Geometry: final body of the model. Coordinates: model frame, mm. A direction names the side the tool comes from. Give positions to 0.01 mm unless a question says otherwise; leave off trailing zeros. Order: outer loops, then holes, each group sorted by start corner. A loop starts at its lowest first (then second) coordinate and runs counter-clockwise, first axis right, second up. Notation, with made-up numbers: M -37.75,28 L 6.25,28 A11 cw 6.25,42 Z; hole C 74.25,68 d11. An arc over 180 degrees is marked long. Write item = value, one per line. Start each with the question number.
from build123d import *
from build123d.topology import SkipClean

# Parameters (mm, degrees)
BOSS_EXTRU_1_START = 5
BOSS_EXTRU_1_DEPTH = 5


with BuildPart() as part:
    # Esquisse1 → Révolution1 (revolve)
    with BuildSketch(Plane(origin=(0, 0, 0), x_dir=(1, 0, 0), z_dir=(0, 1, 0)), mode=Mode.PRIVATE) as r_volution1_sk:
        Polygon((-95.869703244, 5), (-95.869703244, -5), (-78.192033714, -22.67766953), (-78.192033714, -17.67766953), (-81, -14.869703244), (-81, 0), (-87.869703244, 0), (-87.869703244, 5), align=None)
    revolve(r_volution1_sk.sketch.rotate(Axis((0, 0, 0), (0, 0, -1)), 180), axis=Axis((0, 0, 0), (0, 0, -1)))

    # Esquisse6 → Boss.-Extru.1 (add)
    with SkipClean():  # the faces are left unmerged after this step: merging them gives an invalid solid
        with BuildSketch(Plane(origin=(0, 0, 0), x_dir=(-1, 0, 0), z_dir=(0, 0, -1)).offset(BOSS_EXTRU_1_START)):
            with BuildLine():
                Line((80.961410561, -2.5), (87.834132022, -2.5))
                ThreePointArc((87.834132022, -2.5), (87.869703244, 0), (87.834132022, 2.5))
                Line((87.834132022, 2.5), (80.961410561, 2.5))
                ThreePointArc((80.961410561, 2.5), (81, 0), (80.961410561, -2.5))
            make_face()
        boss_extru_1 = extrude(amount=-BOSS_EXTRU_1_DEPTH)

    # Symétrie1: Boss.-Extru.1 across plane
    add(boss_extru_1.mirror(Plane(origin=(0, 0, 0), x_dir=(0, 0, 1), z_dir=(1, 0, 0))))


solid = part.part
1) Cut plane B-B (y = 0). Return loops of the section in (x, z), plus the area to 3 significant figures.
2) Access query for faces 1 (the cylindrical face through (1.9, -87.85, -2.54)), 2 (the cylindrical face through (-20.78, 93.59, 0.07)). Directions: +Z, -Z, +X, -X, +Y, -Y. A direction counts if a zero-diameter tool reaches every point of the face in a straight line with its end or side. Return the directions, or none.
3) Cut plane C-C (z = 12.5). Return loops of the section in (x, y), plus the area to 3 significant figures.
4) Cut plane A-A (x = 0). Return loops of the section in (y, z).
5) Ray query, L1, parallel to Y at x = 59, z = 14.75; L2, parallel to X at y = 26, z = 20.75; L3, parallel to Y at x = -7, z = 10. Return the intervals inside material, ascending.
6) Draft query along Y for faces 3 (the cylindrical face through (-1.9, 87.85, -2.54)), 4 (the conical face through (-17.1, 77.2, 21.8)), 5 (the flat face through (84, -2.5, -3)), 6 (the flat face through (85, 0, -5)). Return one class per face: pulls with the +Y half, pulls with the -Y half, needs draft (parallel to the pull), parting line crosses it, or undercut.
7) Pin query (flat end, axial travel): pin 1 Ø2 at (y, z) = (63, -1.5) entering from -X; pin 2 Ø1.5 at (x, z) = (-83, -3) entering from +Y; pin 3 Ø1 at (x, z) = (-29, 8) entering from -Y; pin 4 Ø6 at (x, y) = (-68, -72.5) entering from +Z. Return the tip coordinate at first contact, or that it passes through.
Reply:
q1.outline = M -95.87,-5 L -81,-5 L -81,14.87 L -78.19,17.68 L -78.19,22.68 L -95.87,5 Z; M 78.19,17.68 L 81,14.87 L 81,-5 L 95.87,-5 L 95.87,5 L 78.19,22.68 Z
q1.area = 547 mm²
q2.face_1 = -Z
q2.face_2 = +Z, -Z
q3.outline = C 0,0 d176.74; hole C 0,0 d162
q3.area = 3,920 mm²
q4.outline = M -95.87,-5 L -87.87,-5 L -87.87,0 L -81,0 L -81,14.87 L -78.19,17.68 L -78.19,22.68 L -95.87,5 Z; M 78.19,17.68 L 81,14.87 L 81,0 L 87.87,0 L 87.87,-5 L 95.87,-5 L 95.87,5 L 78.19,22.68 Z
q5.L1 = -62.73 to -55.5, 55.5 to 62.73
q5.L2 = -75.78 to -73.74, 73.74 to 75.78
q5.L3 = -90.6 to -80.7, 80.7 to 90.6
q6.face_3 = undercut
q6.face_4 = parting line crosses it
q6.face_5 = undercut
q6.face_6 = needs draft
q7.pin_1 = -73.12
q7.pin_2 = 49.25
q7.pin_3 = -88.78
q7.pin_4 = through
